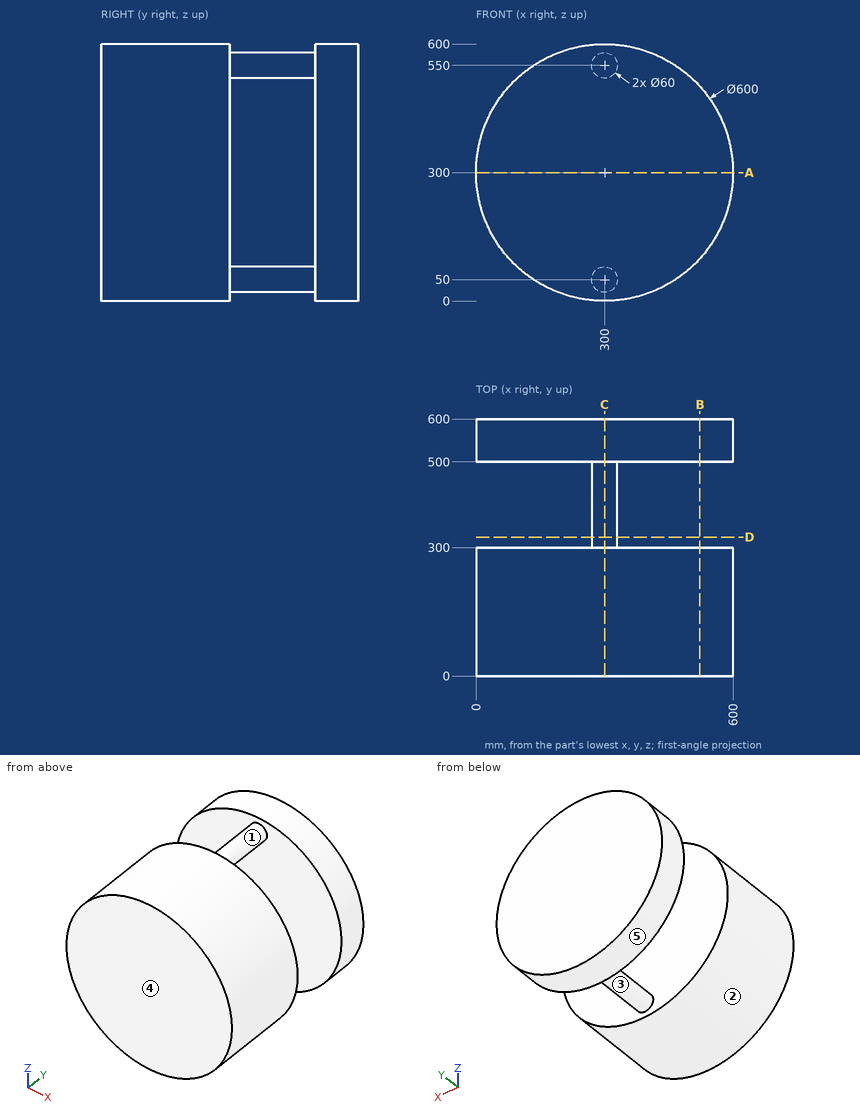
Verification items for this drawing (mm, ordinates from the low corner). A direction names the side the tool comes from. Round coordinates to 2 decimals unless told otherwise and drop trailing zeros. Loops run counter-clockwise (first coordinate to the right, second up) from the corner with the lowest first, then second, coordinate; pieces in that order, holes last. Notation, with made-up numbers: (76, 75) -> (104, 75) arc R19 ccw to (104, 103) -> close; hole circle Ø8 at (54, 28). An arc over 180 degrees is marked (long way). Write item = value, one per line. Start each with the question number.
1) Sectioned sample at B-B, the plane x = 522.5. Record the cut outline in (y, z), plus the area to 3 significant figures.
2) Thickness scan on probe 1 along Y at (x, z) = (232, 147); probe 2 along Z at (x, y) = (292.5, 345); probe 3 along Z at (x, y) = (300.5, 201.5). Record the ranges inside material, lowest first.
3) Set-up check for the marked faces 1 and 2: record each of +Z, -Z, +X, -X, +Y, -Y from which the full face is reachable in a straight line by a thin tool's end or side.
4) Release check for a two-part mould opening along Z. For the marked faces 3, 4 and 5 record: released by +Z, released by -Z, zero draft, split by the parting line, or undercut.
5) Sectioned sample at A-A, the plane z = 300. Record the cut outline in (x, y).
6) Sectioned sample at C-C, the plane x = 300. Record the cut outline in (y, z), plus the area to 3 significant figures.
7) Sectioned sample at D-D, the plane y = 324.5. Record the cut outline in (x, z).
8) Gauge pin test, flat ends, axial feed: pin 1 Ø8 at (x, y) = (192.5, 127.5) entering from +Z; pin 2 Ø5 at (x, y) = (202, 219) entering from -Z; pin 3 Ø3 at (x, y) = (189.5, 106.5) entering from -Z. Record the tip position at first contact, or that the pin passes through.
Results are:
q1.outline = (0, 98.77) -> (300, 98.77) -> (300, 501.23) -> (0, 501.23) -> close; (500, 98.77) -> (600, 98.77) -> (600, 501.23) -> (500, 501.23) -> close
q1.area = 161,000 mm^2
q2.probe_1 = 0 to 300, 500 to 600
q2.probe_2 = 20.95 to 79.05, 520.95 to 579.05
q2.probe_3 = 0 to 600
q3.face_1 = none
q3.face_2 = +Y, -Y
q4.face_3 = undercut
q4.face_4 = zero draft
q4.face_5 = split by the parting line
q5.outline = (0, 0) -> (600, 0) -> (600, 300) -> (0, 300) -> close; (0, 500) -> (600, 500) -> (600, 600) -> (0, 600) -> close
q6.outline = (0, 0) -> (300, 0) -> (300, 20) -> (500, 20) -> (500, 0) -> (600, 0) -> (600, 600) -> (500, 600) -> (500, 580) -> (300, 580) -> (300, 600) -> (0, 600) -> close; hole (300, 80) -> (500, 80) -> (500, 520) -> (300, 520) -> close
q6.area = 264,000 mm^2
q7.outline = circle Ø60 at (300, 50); circle Ø60 at (300, 550)
q8.pin_1 = 581.58
q8.pin_2 = 15.61
q8.pin_3 = 20.5
